Here's how the part is built. I have some questions about the finished solid (model axes, mm). Face numbers are marked on the shaded views. A direction names the side the tool comes from. Round coordinates to 2 decimals unless told otherwise and drop trailing zeros. Loops run counter-clockwise (first coordinate to the right, second up) from the corner with the lowest first, then second, coordinate; pieces in that order, holes last. Notation, with made-up numbers: M 8,61 L 43,61 A28 ccw 43,94 Z; hole C -26,31 d5. An arc over 180 degrees is marked long. Use a Markdown table: item, result.
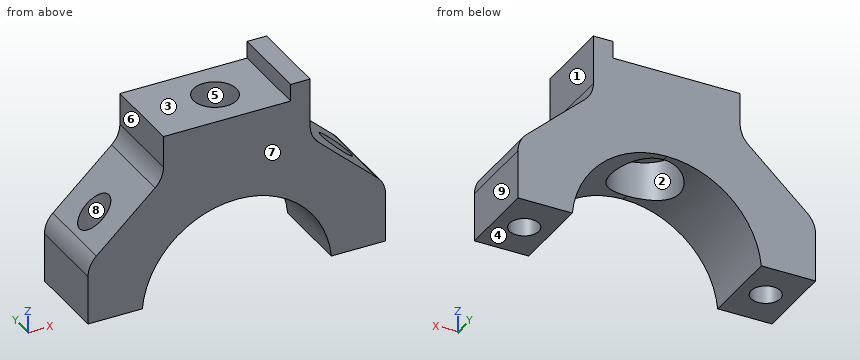
from build123d import *

# Parameters (mm, degrees)
F1_DEPTH  = 9.5
F2_R      = 3.4
F3_DEPTH  = 23.0524285714
F5_W      = 29.5
F5_H      = 19
F6_DEPTH  = 4
F7_R      = 8
F8_DEPTH  = 40.001
F9_R      = 8
F9_R_2    = 5
F10_DEPTH = 11.5
F11_R     = 6


with BuildPart() as f1:
    # F0 (on Front) → F1 (new body, symmetric)
    with BuildSketch(Plane.XZ):
        with BuildLine():
            Line((-34.5, 2), (-21.9089023002, 2))
            ThreePointArc((-21.9089023002, 2), (-14.8323969742, 16.2480768093), (0, 22))
            Line((0, 22), (0, 46))
            Line((0, 46), (-17, 46))
            Line((-17, 46), (-17, 32))
            Line((-17, 32), (-34.5, 16))
            Line((-34.5, 16), (-34.5, 2))
        make_face()
    extrude(amount=F1_DEPTH, both=True)

    # F2 (on face) → F3 (cut, through all)
    with BuildSketch(Plane(origin=(0, 0, 2), x_dir=(1, 0, 0), z_dir=(0, 0, -1))):
        with Locations((-28, 0)):
            Circle(F2_R)
    extrude(amount=-F3_DEPTH, mode=Mode.SUBTRACT)

    # F4: F1 across plane


with BuildPart() as f1_1:
    add(f1.part)
    add(f1.part.mirror(Plane.YZ))

    # F5 (on face) → F6 (cut)
    with BuildSketch(Plane.XY.offset(46)):
        with Locations((-2.25, 0)):
            Rectangle(F5_W, F5_H)
    extrude(amount=-F6_DEPTH, mode=Mode.SUBTRACT)

    # F7 (on face) → F8 (cut, through all)
    with BuildSketch(Plane.XY.offset(42)):
        Circle(F7_R)
    extrude(amount=-F8_DEPTH, mode=Mode.SUBTRACT)

    # F9 (on face) → F10 (join)
    with BuildSketch(Plane.XY.offset(42)):
        Circle(F9_R)
        Circle(F9_R_2, mode=Mode.SUBTRACT)
    extrude(amount=-F10_DEPTH)

    # F11
    f11_edges = [f1_1.edges().sort_by_distance(p)[0] for p in [
        (-34.5, 0, 16),
        (34.5, 0, 16),
        (-17, 0, 32),
        (17, 0, 32),
    ]]
    fillet(f11_edges, radius=F11_R)


solid = f1_1.part
1. Imagine slicing it at C-C, the plane x = -28. Write out the boundary of the cut face in (y, z), then the cut area to 3 significant figures.
Answer sheet:
| item | result |
|---|---|
| outline | M -9.5,2 L -3.4,2 L -3.4,21.94 L -9.5,21.94 Z; M 3.4,2 L 9.5,2 L 9.5,21.94 L 3.4,21.94 Z |
| area | 243 mm2 |
2. I need wall thicknesses on probe 1 along Y at (x, z) = (28, 9.75); probe 2 along X at (y, z) = (0, 8.75); probe 3 along X at (y, z) = (-2.75, 11.5) (3 decimals). Which ranges of each line are inside material? Lowest first, please. Write a range as from..to.
Answer sheet:
| item | result |
|---|---|
| probe 1 | -9.5..-3.4, 3.4..9.5 |
| probe 2 | -34.5..-31.4, -24.6..-20.19, 20.19..24.6, 31.4..34.5 |
| probe 3 | -34.5..-29.999, -26.001..-18.755, 18.755..26.001, 29.999..34.5 |
3. For pin 1 Ø8 at (y, z) = (2, 16) entering from +X; pin 2 Ø5.5 at (x, y) = (-3, 3.5) entering from +Z; pin 3 Ø8 at (x, y) = (-1, -0.5) entering from -Z; pin 4 Ø4 at (y, z) = (-5.5, 35.5) entering from -X, each with a flat end and sliding along its axis, tell me the tip position at first contact or that it passes through.
Answer sheet:
| item | result |
|---|---|
| pin 1 | x = 34.5 |
| pin 2 | z = 42 |
| pin 3 | z = 30.5 |
| pin 4 | x = -17.11 |
4. We'd pull the mould along X, two halves only. Please class the marked faces 6, 7, 8 and 9: +X half, -X half, draft (parallel to the pull), parting line (faces both ways), or undercut.
Answer sheet:
| item | result |
|---|---|
| face 6 | -X half |
| face 7 | draft |
| face 8 | undercut |
| face 9 | +X half |
5. Imagine slicing it at A-A, the plane z = 10. Write out the boundary of the cut face in (x, y).
Answer sheet:
| item | result |
|---|---|
| outline | M -34.5,-9.5 L -19.6,-9.5 L -19.6,9.5 L -34.5,9.5 Z; M 19.6,-9.5 L 34.5,-9.5 L 34.5,9.5 L 19.6,9.5 Z; hole C -28,0 d6.8; hole C 28,0 d6.8 |
6. Imagine slicing it at D-D, the plane z = 40.5. Write out the boundary of the cut face in (x, y).
Answer sheet:
| item | result |
|---|---|
| outline | M -17,-9.5 L 17,-9.5 L 17,9.5 L -17,9.5 Z; hole C 0,0 d10 |
7. Imagine slicing it at B-B, the plane y = 0. State how many separate pieces and enclosed holes the cut face has, then the cut area to 3 significant figures.
Answer sheet:
| item | result |
|---|---|
| separate pieces | 4 |
| enclosed holes | 0 |
| area | 945 mm2 |
8. Which directions (+Z, -Z, +X, -X, +Y, -Y) give clear straight access to the entire face, cutting with the end or side of a thin tool? Please do the marked faces 1, 2, 3, 4 and 5.
Answer sheet:
| item | result |
|---|---|
| face 1 | +Z, +X, +Y, -Y |
| face 2 | -Z |
| face 3 | +Z, -X, +Y, -Y |
| face 4 | -Z, +X, -X, +Y, -Y |
| face 5 | +Z, -Z |
